Input: dimensioned drawing with shaded views. Units: mm. Origin: part minimum x, y, z. Round coordinates to 2 decimals unless told otherwise and drop trailing zeros. Order: outer loops, then holes, each group sorted by start corner. A loop starts at its lowest first (then second) coordinate and runs counter-clockwise, first axis right, second up. Notation, with made-up numbers: (74, 23) - (107, 23) arc R17 ccw to (107, 44) - close; hole circle Ø5 at (67.25, -16.5). An arc over 180 degrees is marked (long way). Put each result on its own line as item: value. Start each with the question number.
(1) Pull-direction query (Y, two-part tool) for the marked faces 1, 2, 3 and 4; classes: released by +Y, released by -Y, zero draft, split by the parting line, or undercut.
(2) Section C-C (y = 20.25). Output: boundary loops of the cut face in (x, z), and give its area (3 significant figures).
(3) Section A-A (x = 20.25). Output: boundary loops of the cut face in (y, z), and give its area (3 significant figures).
(4) Section D-D (z = 4). Output: boundary loops of the cut face in (x, y).
(5) Pin query (flat end, axial travel): P1, Ø2, axis at x = 29, z = 5.5, coming from the -Y side; P2, Ø19.5, axis at x = 20.25, y = 20.25, coming from the -Z side; P3, Ø7, axis at x = 36.5, y = 20.25, coming from the +Z side. Return the tip coordinate at first contact, or that it passes through.
(6) Material intervals for L1, parallel to X at y = 18.5, z = 5.25; L2, parallel to Y at x = 12.5, z = 4.75; L3, parallel to Y at x = 4, z = 2.5, sorted ascending. Write a range as [from, to].
(7) Section B-B (y = 26.5). Output: boundary loops of the cut face in (x, z).
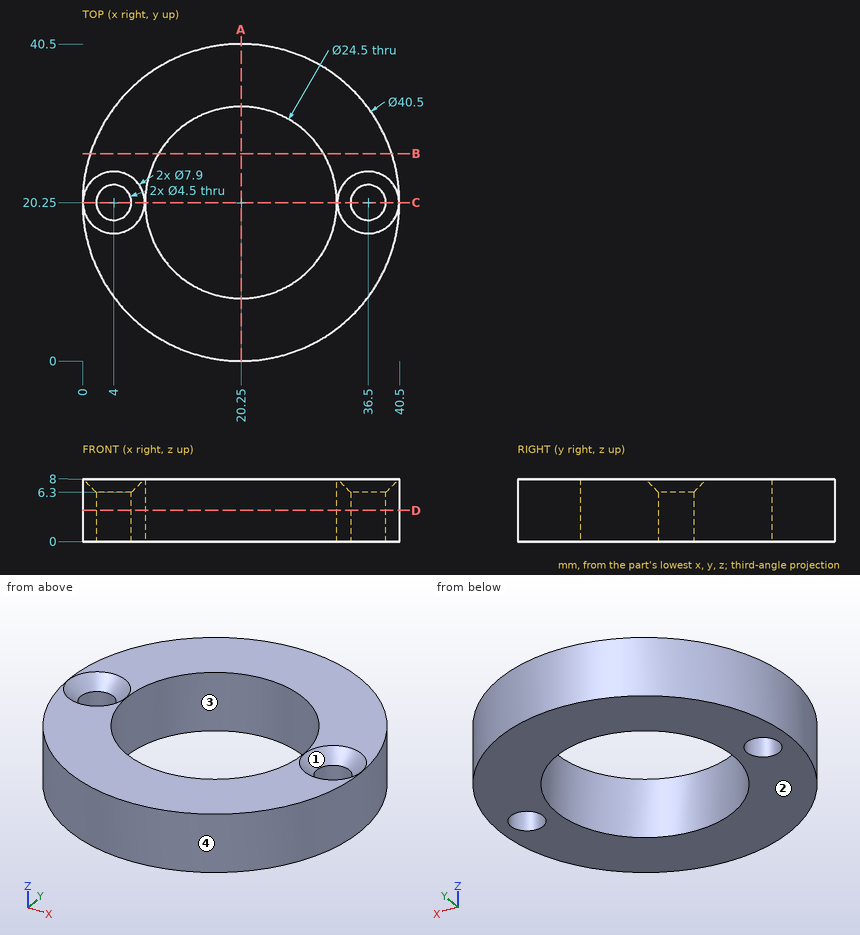
Checks:
1. face 1: undercut
1. face 2: zero draft
1. face 3: undercut
1. face 4: split by the parting line
2. outline: (0, 0) - (1.75, 0) - (1.75, 6.3) - (0.05, 8) - (0, 8) - close; (6.25, 0) - (8, 0) - (8, 8) - (7.95, 8) - (6.25, 6.3) - close; (32.5, 0) - (34.25, 0) - (34.25, 6.3) - (32.55, 8) - (32.5, 8) - close; (38.75, 0) - (40.5, 0) - (40.5, 8) - (40.45, 8) - (38.75, 6.3) - close
2. area: 50.2 mm²
3. outline: (0, 0) - (8, 0) - (8, 8) - (0, 8) - close; (32.5, 0) - (40.5, 0) - (40.5, 8) - (32.5, 8) - close
3. area: 128 mm²
4. outline: circle Ø40.5 at (20.25, 20.25); hole circle Ø4.5 at (4, 20.25); hole circle Ø24.5 at (20.25, 20.25); hole circle Ø4.5 at (36.5, 20.25)
5. P1: stops at y = 1.54
5. P2: passes through
5. P3: stops at z = 7.55
6. L1: x = [0.08, 2.59], [5.41, 8.13], [32.37, 35.09], [37.91, 40.42]
6. L2: y = [1.54, 10.76], [29.74, 38.96]
6. L3: y = [8.17, 18], [22.5, 32.33]
7. outline: (0.99, 0) - (9.71, 0) - (9.71, 8) - (0.99, 8) - close; (30.79, 0) - (39.51, 0) - (39.51, 8) - (30.79, 8) - close
